Verification items for this drawing (mm, ordinates from the low corner). A direction names the side the tool comes from. Round coordinates to 2 decimals unless told otherwise and drop trailing zeros. Loops run counter-clockwise (first coordinate to the right, second up) from the corner with the lowest first, then second, coordinate; pieces in that order, holes last. Notation, with made-up numbers: (25, 36.5) - (31, 36.5) arc R27 ccw to (31, 54.5) - close; hole circle Ø3 at (21, 58.25). An arc over 180 degrees is marked (long way). Use a Markdown table: item, result. Add a question column.
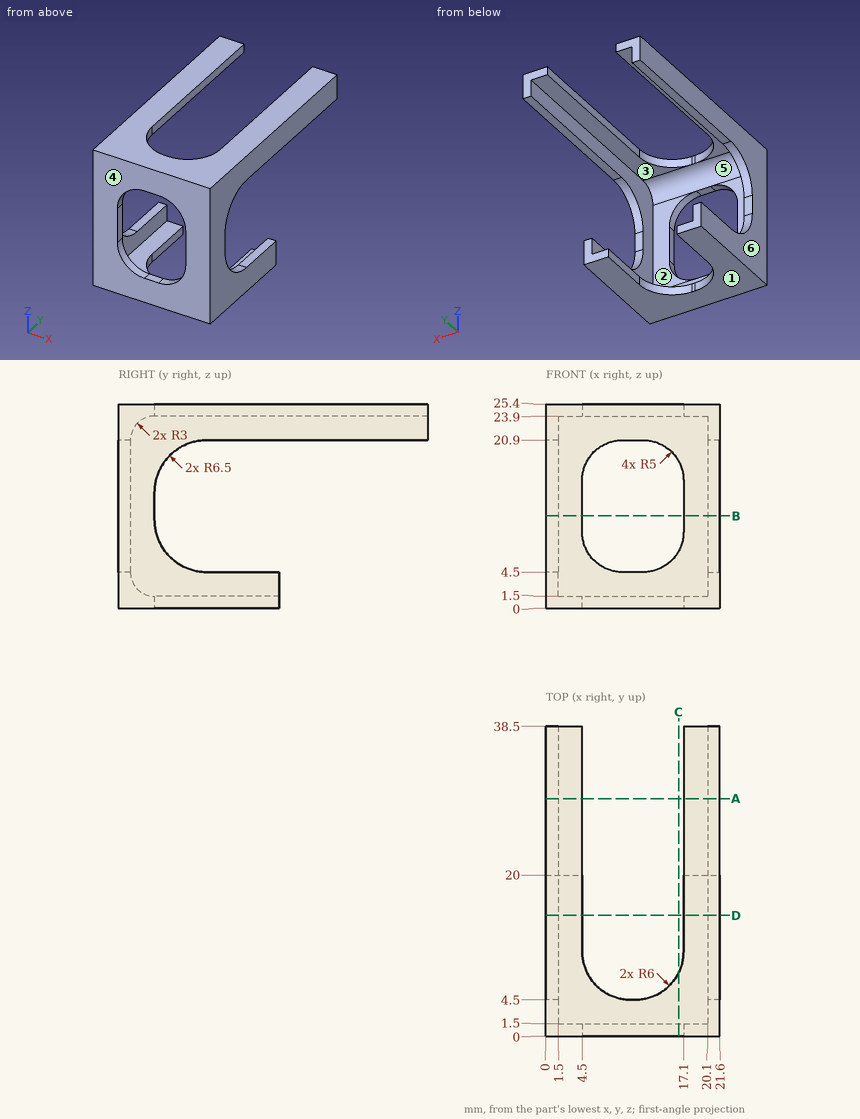
Q1. Section check D-D on y = 15. Record the cut outline in (x, z).
Q2. Release check for a two-part mould opening along X. For the marked faces 3, 4, 5 and 6 record: +X half, -X half, draft (parallel to the pull), parting line (faces both ways), or undercut.
Q3. Section check B-B on z = 11.5. Record the cut outline in (x, y).
Q4. Go/stop test with flat-tipped pins: pin 1 Ø0.5 at (x, z) = (21, 13) entering from +Y; pin 2 Ø1.2 at (x, y) = (1, 31.5) entering from -Z; pin 3 Ø12 at (x, z) = (12, 12) entering from +Y. Record where each tip stops, or that it passes through.
Q5. Section check A-A on y = 29.5. Record the cut outline in (x, z), plus the area to 3 significant figures.
Q6. Thickness scan on line 1 along X through (y, z) = (32, 23.75); line 2 along Z through (x, y) = (2, 18.5); line 3 along Y through (x, z) = (1, 13.5). Record the ranges inside material, lowest first.
Q7. Set-up check for the marked faces 1 and 2: record each of +Z, -Z, +X, -X, +Y, -Y from which the full face is reachable in a straight line by a thin tool's end or side.
Q8. Section check C-C on x = 16.5. Record the cut outline in (y, z) (1 decimal), plus the area to 3 significant figures.
Determined:
| question | item | result |
|---|---|---|
| 1 | outline | (0, 0) - (4.5, 0) - (4.5, 1.5) - (1.5, 1.5) - (1.5, 4.5) - (0, 4.5) - close; (0, 20.9) - (1.5, 20.9) - (1.5, 23.9) - (4.5, 23.9) - (4.5, 25.4) - (0, 25.4) - close; (17.1, 0) - (21.6, 0) - (21.6, 4.5) - (20.1, 4.5) - (20.1, 1.5) - (17.1, 1.5) - close; (17.1, 23.9) - (20.1, 23.9) - (20.1, 20.9) - (21.6, 20.9) - (21.6, 25.4) - (17.1, 25.4) - close |
| 2 | face 3 | undercut |
| 2 | face 4 | draft |
| 2 | face 5 | undercut |
| 2 | face 6 | -X half |
| 3 | outline | (0, 0) - (4.5, 0) - (4.5, 1.5) - (1.5, 1.5) - (1.5, 4.5) - (0, 4.5) - close; (17.1, 0) - (21.6, 0) - (21.6, 4.5) - (20.1, 4.5) - (20.1, 1.5) - (17.1, 1.5) - close |
| 4 | pin 1 | stops at y = 4.5 |
| 4 | pin 2 | stops at z = 20.9 |
| 4 | pin 3 | stops at y = 1.5 |
| 5 | outline | (0, 20.9) - (1.5, 20.9) - (1.5, 23.9) - (4.5, 23.9) - (4.5, 25.4) - (0, 25.4) - close; (17.1, 23.9) - (20.1, 23.9) - (20.1, 20.9) - (21.6, 20.9) - (21.6, 25.4) - (17.1, 25.4) - close |
| 5 | area | 22.5 mm² |
| 6 | line 1 | x = 0 to 1.5, 20.1 to 21.6 |
| 6 | line 2 | z = 0 to 1.5, 23.9 to 25.4 |
| 6 | line 3 | y = 0 to 4.5 |
| 7 | face 1 | -Z, +X, -X, +Y, -Y |
| 7 | face 2 | +Y |
| 8 | outline | (0, 0) - (7.9, 0) - (7.9, 1.5) - (4.5, 1.5) arc R3 cw to (1.5, 4.5) - (1.5, 7.1) - (0, 7.1) - close; (0, 18.3) - (1.5, 18.3) - (1.5, 20.9) arc R3 cw to (4.5, 23.9) - (7.9, 23.9) - (7.9, 25.4) - (0, 25.4) - close |
| 8 | area | 44.4 mm² |
